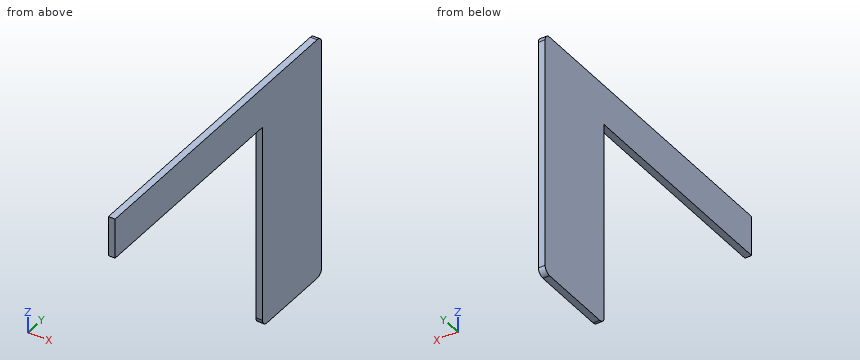
from build123d import *

# Parameters (mm, degrees)
EXTRUDE_1_DEPTH = 0.3
FILLET_1_R      = 0.3
SKETCH_4_W      = 0.3
SKETCH_4_H      = 1.8
EXTRUDE_3_DEPTH = 3


with BuildPart() as part:
    # 草图1 → 凸台-拉伸1 (new body)
    with BuildSketch(Plane(origin=(0, 0, 0), x_dir=(0, 0, -1), z_dir=(1, 0, 0))):
        Polygon((-5.5, -2), (-5.5, -1.5), (-5.5, -0.5), (-5.5, 0.5), (-5.5, 1.5), (-5.5, 2), (5.5, 2), (5.5, 1.5), (5.5, 0.5), (5.5, -0.5), (5.5, -1.5), (5.5, -2), (-3.7, -2), (-3.7, -8.98), (-5.5, -8.98), align=None)
    extrude(amount=EXTRUDE_1_DEPTH)

    # 圆角1
    fillet_1_edges = [part.edges().sort_by_distance(p)[0] for p in [
        (0.15, -2, -5.5),
        (0.15, 2, 5.5),
        (0.15, 2, -5.5),
    ]]
    fillet(fillet_1_edges, radius=FILLET_1_R)

    # 草图4 → 凸台-拉伸3 (add)
    with BuildSketch(Plane.XZ.offset(8.98)):
        with Locations((0.15, 4.6)):
            Rectangle(SKETCH_4_W, SKETCH_4_H)
    extrude(amount=EXTRUDE_3_DEPTH)


solid = part.part
CAD build for the part. Positions are in the model's coordinates, mm. Coordinates: 2 decimals unless noted, no trailing zeros. Loops run counter-clockwise (first coordinate to the right, second up) from the corner with the lowest first, then second, coordinate; pieces in that order, holes last. Notation, with made-up numbers: (70.5, -17.75) - (115.5, -17.75) arc R22 cw to (115.5, 13.25) - close; hole circle Ø10 at (58, 86.25). An arc over 180 degrees is marked (long way). Write item = value, one per line. Start each with the question number.
Q1. Cut at A-A, the plane x = 0.05. List the corners of the cut face in (y, z).
Q2. Cut at C-C, the plane y = -10.25. List the corners of the cut face in (x, z), then the cut area to 3 significant figures.
Q3. Cut at B-B, the plane z = 1.5. List the corners of the cut face in (x, y).
Q4. Drill centre lines: L1, parallel to Y at x = 0.25, z = 1; L2, parallel to Z at x = 0.1, y = -6.5. Where is each one in solid material? Low to high.
Computed:
q1.outline = (-11.98, 3.7) - (-2, 3.7) - (-2, -5.2) arc R0.3 ccw to (-1.7, -5.5) - (1.7, -5.5) arc R0.3 ccw to (2, -5.2) - (2, 5.2) arc R0.3 ccw to (1.7, 5.5) - (-11.98, 5.5) - close
q2.outline = (0, 3.7) - (0.3, 3.7) - (0.3, 5.5) - (0, 5.5) - close
q2.area = 0.540 mm²
q3.outline = (0, -2) - (0.3, -2) - (0.3, 2) - (0, 2) - close
q4.L1 = -2 to 2
q4.L2 = 3.7 to 5.5
